from build123d import *

# Parameters (mm, degrees)
F0_W     = 200
F0_H     = 100
F0_R     = 4
F0_R_2   = 11
F0_R_3   = 2
F1_DEPTH = 10
F0_R_4   = 7
F2_DEPTH = 3


with BuildPart() as f1:
    # F0 (on Top) → F1 (new body)
    with BuildSketch(Plane.XY):
        with Locations((-36.014734, 12.836266)):
            Rectangle(F0_W, F0_H)
        with Locations((-116.014734, -25.163734)):
            Circle(F0_R, mode=Mode.SUBTRACT)
        with Locations((-92.014734, -25.163734)):
            Circle(F0_R, mode=Mode.SUBTRACT)
        with Locations((-68.014734, -25.163734)):
            Circle(F0_R, mode=Mode.SUBTRACT)
        with Locations((-16.014734, -17.163734)):
            Circle(F0_R_2, mode=Mode.SUBTRACT)
        with Locations((-126.014734, 12.836266)):
            Circle(F0_R_3, mode=Mode.SUBTRACT)
        with Locations((-116.014734, 12.836266)):
            Circle(F0_R, mode=Mode.SUBTRACT)
        with Locations((-92.014734, 12.836266)):
            Circle(F0_R, mode=Mode.SUBTRACT)
        with Locations((-68.014734, 12.836266)):
            Circle(F0_R, mode=Mode.SUBTRACT)
        with Locations((-116.014734, 50.836266)):
            Circle(F0_R, mode=Mode.SUBTRACT)
        with Locations((-92.014734, 50.836266)):
            Circle(F0_R, mode=Mode.SUBTRACT)
        with Locations((-68.014734, 50.836266)):
            Circle(F0_R, mode=Mode.SUBTRACT)
        with Locations((-36.014734, 12.836266)):
            Circle(F0_R_3, mode=Mode.SUBTRACT)
        with Locations((53.985266, 12.836266)):
            Circle(F0_R_3, mode=Mode.SUBTRACT)
        with Locations((43.985266, 42.836266)):
            Circle(F0_R_2, mode=Mode.SUBTRACT)
    extrude(amount=F1_DEPTH)

    # F0 (on Top) → F2 (join)
    with BuildSketch(Plane.XY):
        with Locations((-16.014734, -17.163734)):
            Circle(F0_R_2)
        with Locations((-16.014734, -17.163734)):
            Circle(F0_R_4, mode=Mode.SUBTRACT)
        with Locations((43.985266, 42.836266)):
            Circle(F0_R_2)
        with Locations((43.985266, 42.836266)):
            Circle(F0_R_4, mode=Mode.SUBTRACT)
    extrude(amount=F2_DEPTH)


solid = f1.part
Could you check a few things on this model? Use its own coordinates, in mm. A direction names the side the tool comes from. Round coordinates to 2 decimals unless told otherwise and drop trailing zeros. Order: outer loops, then holes, each group sorted by start corner. A loop starts at its lowest first (then second) coordinate and runs counter-clockwise, first axis right, second up.
(1) Please list where these lines run through material, in increasing order: line 1 along X through (y, z) = (-27, 2); line 2 along X through (y, z) = (16, 9.25); line 3 along X through (y, z) = (44, 6).
Response values:
line 1: x = -136.01 to -119.57, -112.46 to -95.57, -88.46 to -71.57, -64.46 to 63.99
line 2: x = -136.01 to -118.46, -113.57 to -94.46, -89.57 to -70.46, -65.57 to 63.99
line 3: x = -136.01 to 33.05, 54.92 to 63.99
(2) Imagine slicing it at A-A (x = 44). Write out the boundary of the cut face in (y, z), plus the area to 3 significant figures.
Response values:
outline: (-37.16, 0) - (35.84, 0) - (35.84, 3) - (31.84, 3) - (31.84, 10) - (-37.16, 10) - close; (49.84, 0) - (62.84, 0) - (62.84, 10) - (53.84, 10) - (53.84, 3) - (49.84, 3) - close
area: 804 mm2
(3) If we mould it in two halves opening along X, with no side actions, what happens to faces 1 (the flat face through (-37, 25, 10)), 2 (the cylindrical face through (-96.01, 13.01, 4.93)), 3 (the flat face through (-136.015, 12, 5))? For each: released by +X, released by -X, zero draft, split by the parting line, or undercut.
Response values:
face 1: zero draft
face 2: undercut
face 3: released by -X
(4) Imagine slicing it at B-B (z = 1.5). Count the separate pieces of the cut face and the enclosed holes in it, plus the area to 3 significant figures.
Response values:
separate pieces: 1
enclosed holes: 14
area: 19,200 mm2
(5) I'm going to push flat-ended pins straight in: pin 1 (6.5 mm diameter, centred on x = -92.01, y = 12.84, fed in from +Z); pin 2 (10.5 mm diameter, centred on x = -116.01, y = 50.84, fed in from +Z); pin 3 (6.5 mm diameter, centred on x = -19.5, y = -19, fed in from +Z). Where does each tip first touch, or does it pass through?
Response values:
pin 1: passes through
pin 2: stops at z = 10
pin 3: stops at z = 3
(6) Which directions (+Z, -Z, +X, -X, +Y, -Y) give clear straight access to the entire face, cutting with the end or side of a thin tool? Please do faces 4 (the flat face through (43.83, 35.66, 3)), 5 (the cylindrical face through (-120.01, 51.01, 4.93)).
Response values:
face 4: +Z
face 5: +Z, -Z
